Design review of the part built by this model. Coordinates are the model's own, in mm. Coordinates: 2 decimals unless noted, no trailing zeros. Loops run counter-clockwise (first coordinate to the right, second up) from the corner with the lowest first, then second, coordinate; pieces in that order, holes last. Notation, with made-up numbers: M 57,-37 L 90,-37 A11 ccw 90,-24 Z; hole C -15.5,89 d5. An arc over 180 degrees is marked long. Put each result on its own line as item: value. Start each with the question number.
(1) Clearance check with flat-ended pins moving along their axes: pin 1 (6 mm diameter, centred on y = 11, z = 65.5, fed in from -X); pin 2 (2.5 mm diameter, centred on y = 6.35, z = 77.79, fed in from +X). State where each tip first meets the part, or that it passes through.
(2) Take a section at B-B, the plane x = 1.25. Give the boundary of the cut face in (y, z).
(3) Take a section at A-A, the plane y = 6.35. Give the boundary of the cut face in (x, z).
(4) For probe 1 along Z at (x, y) = (5.25, 7.25); probe 2 along Y at (x, z) = (5.75, 7.5); probe 3 along Z at (x, y) = (2.5, 8.25), list the stretches that pass through material, from the lowest coordinate up. Write a range as [from, to].
(5) The part is to be moulded in two halves that separate along Z. For faces 1 (the flat face through (0, 6, 53)), 2 (the flat face through (3, 6, 0)), 3 (the cylindrical face through (3.131, 5.275, 10.53)), say which applies: +Z half, -Z half, draft (parallel to the pull), parting line (faces both ways), or undercut.
```python
from build123d import *

# Parameters (mm, degrees)
SKETCH1_W              = 6.35
SKETCH1_H              = 12.7
EXTRUDE1_DEPTH         = 107.95
F_10_CLEARANCE_HOLE1_D = 5.6134
F_6_32_TAPPED_HOLE1_D  = 2.7051


with BuildPart() as part:
    # Sketch1 → Extrude1 (new body)
    with BuildSketch(Plane.XY):
        with Locations((3.175, 6.35)):
            Rectangle(SKETCH1_W, SKETCH1_H)
    extrude(amount=EXTRUDE1_DEPTH)

    # #10 Clearance Hole1 (through all)
    with Locations(Plane(origin=(6.35, 0, 0), x_dir=(0, 0, -1), z_dir=(1, 0, 0))):
        with Locations((-42.8625, 6.35), (-7.9375, 6.35)):
            Hole(F_10_CLEARANCE_HOLE1_D / 2)

    # #6-32 Tapped Hole1 (through all)
    with Locations(Plane.ZY):
        with Locations((100.0125, 6.35), (77.7875, 6.35)):
            Hole(F_6_32_TAPPED_HOLE1_D / 2)


solid = part.part
```
Computed values:
1. pin 1: stops at x = 0
1. pin 2: passes through
2. outline: M 0,0 L 12.7,0 L 12.7,107.95 L 0,107.95 Z; hole C 6.35,7.94 d5.61; hole C 6.35,42.86 d5.61; hole C 6.35,77.79 d2.71; hole C 6.35,100.01 d2.71
3. outline: M 0,0 L 6.35,0 L 6.35,5.13 L 0,5.13 Z; M 0,10.74 L 6.35,10.74 L 6.35,40.06 L 0,40.06 Z; M 0,45.67 L 6.35,45.67 L 6.35,76.43 L 0,76.43 Z; M 0,79.14 L 6.35,79.14 L 6.35,98.66 L 0,98.66 Z; M 0,101.37 L 6.35,101.37 L 6.35,107.95 L 0,107.95 Z
4. probe 1: z = [0, 5.28], [10.6, 40.2], [45.52, 76.78], [78.8, 99], [101.02, 107.95]
4. probe 2: y = [0, 3.58], [9.12, 12.7]
4. probe 3: z = [0, 5.87], [10, 40.8], [44.93, 107.95]
5. face 1: draft
5. face 2: -Z half
5. face 3: undercut
